Read the model definition and answer for the solid it produces. Units are mm, in the model's axes. A direction names the side the tool comes from. Coordinates: 2 decimals unless noted, no trailing zeros. Order: outer loops, then holes, each group sorted by start corner. A loop starts at its lowest first (then second) coordinate and runs counter-clockwise, first axis right, second up. Notation, with made-up numbers: M 75.5,-37.75 L 127.5,-37.75 A28 cw 127.5,-14.75 Z; hole C -6,-18.5 d9. An arc over 180 degrees is marked long. Put each result on its own line as item: value.
from build123d import *

# Parameters (mm, degrees)
F0_W     = 23.4
F0_H     = 52
F1_DEPTH = 2
F3_START = 15.05
F3_DEPTH = 9.95
F4_W     = 4.5600925213
F4_H     = 1.5
F4_W_2   = 8.5201850425
F5_DEPTH = 2.95
F6_START = -16.5
F6_DEPTH = 10.5


with BuildPart() as f1:
    # F0 (on Top) → F1 (new body)
    with BuildSketch(Plane.XY):
        with Locations((0, 1)):
            Rectangle(F0_W, F0_H)
    extrude(amount=F1_DEPTH)

    # F2 (on Front) → F3 (join)
    with BuildSketch(Plane.XZ.offset(F3_START)):
        Polygon((2.2934258546, 4.95), (4.2600925213, 2), (7.1399074787, 2), (9.1065741454, 4.95), align=None)
        Polygon((-4.2600925213, 2), (-2.2934258546, 4.95), (-9.1065741454, 4.95), (-7.1399074787, 2), align=None)
    extrude(amount=F3_DEPTH)

    # F4 (on face) → F5 (join)
    with BuildSketch(Plane.XY.offset(2)):
        with Locations((9.4199537394, -24.25)):
            Rectangle(F4_W, F4_H)
        with Locations((0, -24.25)):
            Rectangle(F4_W_2, F4_H)
        with Locations((-9.4199537394, -24.25)):
            Rectangle(F4_W, F4_H)
    extrude(amount=F5_DEPTH)

    # F2 (on Front) → F6 (join)
    with BuildSketch(Plane.XZ.offset(F6_START)):
        Polygon((2.2934258546, 4.95), (4.2600925213, 2), (7.1399074787, 2), (9.1065741454, 4.95), align=None)
        Polygon((-4.2600925213, 2), (-2.2934258546, 4.95), (-9.1065741454, 4.95), (-7.1399074787, 2), align=None)
    extrude(amount=-F6_DEPTH)


solid = f1.part
Q1. Find section B-B on y = 21. Write down the section's boundary in (x, z), plus the area to 3 significant figures.
Answers below:
outline: M -11.7,0 L 11.7,0 L 11.7,2 L 7.14,2 L 9.11,4.95 L 2.29,4.95 L 4.26,2 L -4.26,2 L -2.29,4.95 L -9.11,4.95 L -7.14,2 L -11.7,2 Z
area: 75.4 mm^2
Q2. Find section D-D on x = -8.5. Write down the section's boundary in (y, z), plus the area to 3 significant figures.
Answers below:
outline: M -25,0 L 27,0 L 27,2 L -23.5,2 L -23.5,4.04 L -15.05,4.04 L -15.05,4.95 L -25,4.95 Z; M 16.5,4.04 L 27,4.04 L 27,4.95 L 16.5,4.95 Z
area: 126 mm^2
Q3. Find section A-A on x = -5. Write down the section's boundary in (y, z).
Answers below:
outline: M -25,0 L 27,0 L 27,4.95 L 16.5,4.95 L 16.5,2 L -15.05,2 L -15.05,4.95 L -25,4.95 Z
Q4. Given pin 1 (7 mm diameter, centred on x = -0.5, y = -3, fed in from +Z); pin 2 (0.9 mm diameter, centred on x = 1.5, z = 3.5, fed in from +Y), each flat-ended and moving along its own axis, determine where each tip first touches the part or whether it passes through.
Answers below:
pin 1: stops at z = 2
pin 2: stops at y = -23.5
Q5. Find section C-C on z = 3.1. Write down the section's boundary in (x, y), plus the area to 3 significant figures.
Answers below:
outline: M -11.7,-25 L 11.7,-25 L 11.7,-23.5 L 7.87,-23.5 L 7.87,-15.05 L 3.53,-15.05 L 3.53,-23.5 L -3.53,-23.5 L -3.53,-15.05 L -7.87,-15.05 L -7.87,-23.5 L -11.7,-23.5 Z; M -7.87,16.5 L -3.53,16.5 L -3.53,27 L -7.87,27 Z; M 3.53,16.5 L 7.87,16.5 L 7.87,27 L 3.53,27 Z
area: 200 mm^2
Q6. For a pull along Y with two mould halves and no side action, classify faces 5 (the face through (0, -25, 2)), 6 (the face through (3.26, -19.22, 3.5)), 7 (the face through (-6, 16.5, 4)) as +Y half, -Y half, draft (parallel to the pull), parting line (faces both ways), or undercut.
Answers below:
face 5: -Y half
face 6: draft
face 7: undercut
Q7. Consider line 1 along Y through (x, z) = (3.75, 3.35); line 2 along Z through (x, y) = (3, 3.5); line 3 along Z through (x, y) = (2.75, -19.5). Determine where each line is inside the solid, lowest interval first.
Answers below:
line 1: y = -25 to -15.05, 16.5 to 27
line 2: z = 0 to 2
line 3: z = 0 to 2, 4.27 to 4.95
Q8. A tool of negligible diameter and unlimited length cuts with its end or side. For faces 1 (the face through (-10, -23.5, 3)), 2 (the face through (0, 2, 2)), 3 (the face through (3.26, 21.68, 3.5)), 4 (the face through (8.109, 21.676, 3.454)), from which of +Z, -Z, +X, -X, +Y, -Y can it reach the whole face along a straight path? Write none if from no direction.
Answers below:
face 1: -X, +Y
face 2: none
face 3: +Y
face 4: +X, +Y
